Source: CAD feature listing. Evaluate the final solid. Frame: model axes, mm. A direction names the side the tool comes from. Round coordinates to 2 decimals unless told otherwise and drop trailing zeros. Loops run counter-clockwise (first coordinate to the right, second up) from the corner with the lowest first, then second, coordinate; pieces in that order, holes last.
Item 1: Section query C-C on x = 1395.5. Return loops of the section in (y, z), then the cut area to 3 significant figures.
Item 2: Section query A-A on z = -364. Return loops of the section in (x, y), then the cut area to 3 significant figures.
Item 3: Section query B-B on y = 376. Return loops of the section in (x, z).
Item 4: First-contact query: P1, Ø8, axis at y = 454, z = -298, coming from the +X side; P2, Ø1, axis at x = 646.5, y = 329, coming from the -Z side; P3, Ø23, axis at x = 407.5, z = -425.5, coming from the +Y side. Flat tips, straight axial feed; report the tip coordinate or a pass-through.
Item 5: Pull-direction query (X, two-part tool) for faces 4 (the flat face through (393, 901.7, -351)), 5 (the cylindrical face through (1495.028, 883.848, 12.522)), 6 (the flat face through (751, 464, 0)); classes: released by +X, released by -X, zero draft, split by the parting line, or undercut.
Item 6: Section query D-D on y = 73.5. Return loops of the section in (x, z).
Item 7: Access query for faces 1 (the flat face through (355.6, 451, -351)), 2 (the flat face through (393, 12.7, -351)), 3 (the flat face through (431.8, 451, -351)). Directions: +Z, -Z, +X, -X, +Y, -Y. A direction counts if a zero-diameter tool reaches every point of the face in a straight line with its end or side. Return the directions, or none.
Item 8: Ray query, L1, parallel to X at y = 503.5, z = -659; L2, parallel to Z at x = 295, y = 862.5; L3, parallel to Y at x = 405, z = -343. Return the intervals inside material, ascending.
```python
from build123d import *

# Parameters (mm, degrees)
F2_DEPTH = 25.4
F1_W     = 76.2
F1_H     = 889
F3_DEPTH = 711.2


with BuildPart() as f2:
    # F0 (on Top) → F2 (new body)
    with BuildSketch(Plane.XY):
        with BuildLine():
            ThreePointArc((0, 101.6), (29.757951, 29.757951), (101.6, 0))
            Line((101.6, 0), (1422.4, 0))
            ThreePointArc((1422.4, 0), (1494.242049, 29.757951), (1524, 101.6))
            Line((1524, 101.6), (1524, 812.8))
            ThreePointArc((1524, 812.8), (1494.242049, 884.642049), (1422.4, 914.4))
            Line((1422.4, 914.4), (101.6, 914.4))
            ThreePointArc((101.6, 914.4), (29.757951, 884.642049), (0, 812.8))
            Line((0, 812.8), (0, 101.6))
        make_face()
    extrude(amount=F2_DEPTH)

    # F1 (on Top) → F3 (join)
    with BuildSketch(Plane.XY):
        with Locations((393.7, 457.2)):
            Rectangle(F1_W, F1_H)
        with Locations((1130.3, 457.2)):
            Rectangle(F1_W, F1_H)
    extrude(amount=-F3_DEPTH)


solid = f2.part
```
Data:
1. outline: (0, 0) - (914.4, 0) - (914.4, 25.4) - (0, 25.4) - close
1. area: 23,200 mm2
2. outline: (355.6, 12.7) - (431.8, 12.7) - (431.8, 901.7) - (355.6, 901.7) - close; (1092.2, 12.7) - (1168.4, 12.7) - (1168.4, 901.7) - (1092.2, 901.7) - close
2. area: 135,000 mm2
3. outline: (0, 0) - (355.6, 0) - (355.6, -711.2) - (431.8, -711.2) - (431.8, 0) - (1092.2, 0) - (1092.2, -711.2) - (1168.4, -711.2) - (1168.4, 0) - (1524, 0) - (1524, 25.4) - (0, 25.4) - close
4. P1: stops at x = 1168.4
4. P2: stops at z = 0
4. P3: stops at y = 901.7
5. face 4: zero draft
5. face 5: released by +X
5. face 6: undercut
6. outline: (3.96, 0) - (355.6, 0) - (355.6, -711.2) - (431.8, -711.2) - (431.8, 0) - (1092.2, 0) - (1092.2, -711.2) - (1168.4, -711.2) - (1168.4, 0) - (1520.04, 0) - (1520.04, 25.4) - (3.96, 25.4) - close
7. face 1: -Z, -X, +Y, -Y
7. face 2: -Z, +X, -X, -Y
7. face 3: -Z, +Y, -Y
8. L1: x = 355.6 to 431.8, 1092.2 to 1168.4
8. L2: z = 0 to 25.4
8. L3: y = 12.7 to 901.7
